Autodesk Inventor part; units mm, degrees
ref_plane "YZ Plane" through (0, 0, 0) normal (1, 0, 0) x (0, 1, 0)
ref_plane "XZ Plane" through (0, 0, 0) normal (0, 1, 0) x (-1, 0, 0)
ref_plane "XY Plane" through (0, 0, 0) normal (0, 0, 1) x (1, 0, 0)
sketch "Sketch1" plane through (0, 0, 0) normal (0, 1, 0) x (-1, 0, 0)
  circle A0 centre (0, 0) radius 15
  line L0 (0, 0) -> (14.7721, 2.6047)
  line L1 (0, 0) -> (15, 0) construction
  line L2 (0, 0) -> (-2.6047, -14.7721)
  line L3 (0, 0) -> (15, 0) construction
  line L4 (15, 0) -> (13.5, 0)
  circle A1 centre (13.5, 0) radius 1.1
  line L5 (0, -15) -> (0, -13.5)
  circle A2 centre (0, -13.5) radius 1.1
  dimension "d0" = 30
  dimension "d1" = 10
  dimension "d2" = 100
  dimension "d3" = 1.5
  dimension "d4" = 2.2
  dimension "d5" = 1.5
  dimension "d6" = 2.2
extrude "Extrusion1" add sketch "Sketch1" along normal blind 4 contours A0 L2 L0 picked at (8.0845, -3.2878)
sketch "Sketch2" plane through (0, 4, 0) normal (0, 1, 0) x (1, 0, 0)
  line L0 (0, 0) -> (2.6047, 14.7721)
  circle A0 centre (0, 0) radius 1
  dimension "d9" = 2
extrude "Extrusion2" cut sketch "Sketch2" against normal blind 4
sketch "Sketch3" plane through (0, 4, 0) normal (0, 1, 0) x (1, 0, 0)
  circle A0 centre (0, 0) radius 2.375
  dimension "d12" = 4.75
extrude "Extrusion3" cut sketch "Sketch3" against normal blind 10
sketch "Sketch4" plane through (0, 4, 0) normal (0, 1, 0) x (1, 0, 0)
  circle A0 centre (0, 0) radius 3.5
  line L0 (0.4124, 2.3389) -> (2.6047, 14.7721)
  circle A1 centre (0, 0) radius 2.375
  dimension "d15" = 7
extrude "Extrusion4" add sketch "Sketch4" against normal blind 4
sketch "Sketch5" plane through (0, 4, 0) normal (0, 1, 0) x (1, 0, 0)
  arc A0 (2.6047, 14.7721) -> (-14.7721, -2.6047) centre (0, 0) ccw
  line L0 (2.6047, 14.7721) -> (3.4935, 0.2133)
  arc A1 (-3.4468, -0.6078) -> (0.6078, 3.4468) centre (0, 0) ccw
  line L1 (-14.7721, -2.6047) -> (-3.4468, -0.6078)
  line L2 (-14.7721, -2.6047) -> (-0.2133, -3.4935)
  line L3 (-14.7721, -2.6047) -> (-3.4468, -0.6078)
  line L4 (0.6078, 3.4468) -> (2.6047, 14.7721)
  line L5 (2.6047, 14.7721) -> (0.6078, 3.4468)
  circle A2 centre (0, 0) radius 3.5
extrude "Extrusion5" add sketch "Sketch5" against normal blind 4 contours L0 A1 L4 | L1 A1 L2
fillet "Fillet1" radius 2 2 edges at (-14.7721, 2, 2.6047) (2.6047, 2, -14.7721)
sketch "Sketch6" plane through (0, 4, 0) normal (0, 1, 0) x (1, 0, 0)
  circle A0 centre (0, 13.5) radius 1.1
  line L0 (-1.1, 13.5) -> (-1.1, 18.6359)
  circle A1 centre (-13.5, 0) radius 1.1
  line L1 (-13.5, 1.1) -> (-18.0154, 1.1)
  arc A2 (0.8197, 14.9776) -> (-14.9776, -0.8197) centre (0, 0) ccw
  line L2 (-14.9596, 1.1) -> (-1.1, 14.9596)
  line L3 (-1.1, 14.9596) -> (-5.2086, 18.0633)
  line L4 (-5.2086, 18.0633) -> (-18.2073, 3.056)
  line L5 (-18.2073, 3.056) -> (-14.9596, 1.1)
extrude "Extrusion6" cut sketch "Sketch6" against normal blind 40 contours L2 A2
fillet "Fillet2" radius 2 2 edges at (-14.9596, 2, -1.1) (-1.1, 2, -14.9596)
properties part number "bell_crank_v1"
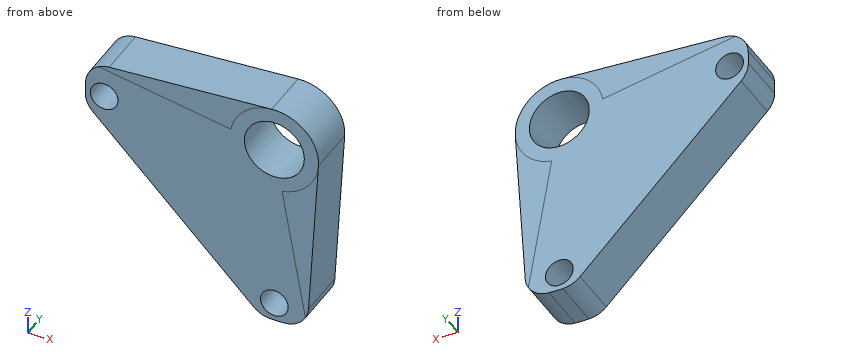
Design review of the part built by this model. Coordinates are the model's own, in mm. Coordinates: 2 decimals unless noted, no trailing zeros. Order: outer loops, then holes, each group sorted by start corner. A loop starts at its lowest first (then second) coordinate and runs counter-clockwise, first axis right, second up. Notation, with made-up numbers: M -9.5,49 L 6.5,49 A12 ccw 6.5,70 Z; hole C 57,77 d10. An arc over 180 degrees is marked long. Answer as a JSON object with one key per item and string values. Group by question number.
1) Add section B-B, the plane y = 1.65. Count the separate pieces of the cut face and the enclosed holes in it, then the cut area to 3 significant figures.
2) Add section C-C, the plane x = 0. Write out the cut boundary in (y, z) (3 decimals).
3) Add section A-A, the plane z = 0. Write out the cut boundary in (x, y) (3 decimals), then the cut area to 3 significant figures.
4) Wall thickness on L1, parallel to Z at x = 0, y = 2.5 (3 decimals); L2, parallel to X at y = 3.15, z = 0.5; L3, parallel to X at y = 0.3, z = 1: over which ranges is each line inside the solid? List them lowest first.
5) Add section D-D, the plane z = -13.5. Write out the cut boundary in (x, y).
6) For pin 1 (1 mm diameter, centred on x = -9, y = 3.5, fed in from +Z); pin 2 (2 mm diameter, centred on y = 1, z = -8.5, fed in from +X); pin 3 (2 mm diameter, centred on x = -3.5, y = 1.5, fed in from -Z), all flat-tipped, find the tip position at first contact; note any pin that passes through.
Computed values:
{
 "1": {"separate pieces": "1", "enclosed holes": "3", "area": "202 mm^2"},
 "2": {"outline": "M 0,-15 L 4,-15 L 4,-14.6 L 0,-14.6 Z; M 0,-12.4 L 4,-12.4 L 4,-2.375 L 0,-2.375 Z; M 0,2.375 L 4,2.375 L 4,3.5 L 0,3.5 Z"},
 "3": {"outline": "M -15,0 L -14.6,0 L -14.6,4 L -15,4 Z; M -12.4,0 L -2.375,0 L -2.375,4 L -12.4,4 Z; M 2.375,0 L 3.5,0 L 3.5,4 L 2.375,4 Z", "area": "46.2 mm^2"},
 "4": {"L1": "z = -15 to -14.6, -12.4 to -2.375, 2.375 to 3.5", "L2": "x = -14.99 to -14.48, -12.52 to -2.32, 2.32 to 3.46", "L3": "x = -14.96 to -13.96, -13.04 to -2.15, 2.15 to 3.35"},
 "5": {"outline": "M -2.56,0 L -1.1,0 L -1.1,4 L -2.56,4 Z; M 1.1,0 L 2.64,0 L 2.64,4 L 1.1,4 Z"},
 "6": {"pin 1": "stops at z = 2.99", "pin 2": "stops at x = 3.05", "pin 3": "stops at z = -13.56"}
}
